Check sheet for the modelled part. Datum: model origin and axes. Units: mm. A direction names the side the tool comes from. Coordinates: 2 decimals unless noted, no trailing zeros. Write each loop counter-clockwise with the first axis right and the second up, starting at its lowest first coordinate (ties: lowest second). Pieces come first, ordered by that corner, then holes. Notation, with made-up numbers: M -19.5,12 L 21.5,12 A10 ccw 21.5,25 Z; hole C 44,-13 d8. An arc over 180 degrees is marked long. Answer as CSV lines item,"result". Start each with the question number.
1) Go/stop test with flat-tipped pins: pin 1 Ø4 at (x, z) = (4, -57.5) entering from +Y; pin 2 Ø1 at (x, y) = (0, -1) entering from +Z; pin 3 Ø0.6 at (x, z) = (0, -37) entering from +Y; pin 4 Ø4 at (x, y) = (3.5, -4) entering from -Z. Record where each tip stops, or that it passes through.
2) Material ranges on L1, parallel to X at y = 0, z = 2.5 (3 decimals); L2, parallel to Z at x = -4.25, y = 1; L3, parallel to X at y = 0.5, z = -12, recorded low to high. Write a range as [from, to].
3) Access from +Z, -Z, +X, -X, +Y, -Y to the whole of each face (thin tool, end or side, straight path). Record for faces 3 (the flat face through (0, 1.568, 3)), 4 (the cylindrical face through (0.328, -1.475, -5.759)), 5 (the flat face through (0, 4.743, -1)).
4) Section check D-D (y = -2.75). Record the cut outline in (x, z), and give its area (3 significant figures).
5) Section check C-C (z = -54.5). Record the cut outline in (x, y).
6) Section check A-A (x = 0). Record the cut outline in (y, z) (3 decimals).
7) Section check B-B (y = 0). Record the cut outline in (x, z) (3 decimals).
8) Draft check along X on faces 1 (the flat face through (1.2, -1.2, -8.89)), 2 (the cylindrical face through (0, -2, 3)). Enter one of: +X half, -X half, draft (parallel to the pull), parting line (faces both ways), or undercut.
from build123d import *

# Parameters (mm, degrees)
BOSS_EXTRUDE1_DEPTH = 6.35
BOSS_EXTRUDE2_START = 2.54
BOSS_EXTRUDE2_DEPTH = 2.54
BOSS_EXTRUDE4_START = 6.35
SKETCH4_R           = 1.5113
BOSS_EXTRUDE4_DEPTH = 6.35
BOSS_EXTRUDE3_DEPTH = 63.5


with BuildPart() as part:
    # Sketch1 → Boss-Extrude1 (new body)
    with BuildSketch(Plane.XY):
        with BuildLine():
            Line((-2.069463106, 4.743200128), (2.069463106, 4.743200128))
            ThreePointArc((2.069463106, 4.743200128), (0, -5.175), (-2.069463106, 4.743200128))
        make_face()
        with BuildLine():
            Line((-1.24126885, 1.568200128), (1.24126885, 1.568200128))
            ThreePointArc((1.24126885, 1.568200128), (0, -2), (-1.24126885, 1.568200128))
        make_face(mode=Mode.SUBTRACT)
    extrude(amount=BOSS_EXTRUDE1_DEPTH)

    # Sketch3 → Boss-Extrude2 (add)
    with BuildSketch(Plane(origin=(0, 0, 0), x_dir=(-1, 0, 0), z_dir=(0, 0, -1)).offset(BOSS_EXTRUDE2_START)):
        with BuildLine():
            Line((-2.069463106, 4.743200128), (2.069463106, 4.743200128))
            ThreePointArc((2.069463106, 4.743200128), (0, -5.175), (-2.069463106, 4.743200128))
        make_face()
    extrude(amount=-BOSS_EXTRUDE2_DEPTH)

    # Sketch4 → Boss-Extrude4 (add)
    with BuildSketch(Plane(origin=(0, 0, -2.54), x_dir=(-1, 0, 0), z_dir=(0, 0, -1)).offset(BOSS_EXTRUDE4_START)):
        with BuildLine():
            Line((2.069463106, 4.743200128), (-2.069463106, 4.743200128))
            ThreePointArc((-2.069463106, 4.743200128), (0, -5.175), (2.069463106, 4.743200128))
        make_face()
        Circle(SKETCH4_R, mode=Mode.SUBTRACT)
    extrude(amount=-BOSS_EXTRUDE4_DEPTH)

    # Sketch2 → Boss-Extrude3 (add)
    with BuildSketch(Plane(origin=(0, 0, -2.54), x_dir=(-1, 0, 0), z_dir=(0, 0, -1))):
        with BuildLine():
            Line((0.997718624, 0.892386667), (-0.997718624, 0.892386667))
            ThreePointArc((-0.997718624, 0.892386667), (0, -1.33858), (0.997718624, 0.892386667))
        make_face()
    extrude(amount=BOSS_EXTRUDE3_DEPTH)


solid = part.part
Results found:
1,pin 1,"passes through"
1,pin 2,"stops at z = 0"
1,pin 3,"stops at y = 0.89"
1,pin 4,"stops at z = -8.89"
2,L1,"x = [-5.175, -2], [2, 5.175]"
2,L2,"z = [-8.89, 6.35]"
2,L3,"x = [-1.24, 1.24]"
3,face 3,"+Z"
3,face 4,"-Z"
3,face 5,"+Z, -Z, +X, -X, +Y"
4,outline,"M -4.38,-8.89 L 4.38,-8.89 L 4.38,6.35 L -4.38,6.35 Z"
4,area,"134 mm2"
5,outline,"M -1,0.89 A1.34 ccw long 1,0.89 Z"
6,outline,"M -5.175,-8.89 L -1.511,-8.89 L -1.511,-2.54 L -1.339,-2.54 L -1.339,-66.04 L 0.892,-66.04 L 0.892,-2.54 L 1.511,-2.54 L 1.511,-8.89 L 4.743,-8.89 L 4.743,6.35 L 1.568,6.35 L 1.568,0 L -2,0 L -2,6.35 L -5.175,6.35 Z"
7,outline,"M -5.175,-8.89 L -1.511,-8.89 L -1.511,-2.54 L -1.339,-2.54 L -1.339,-66.04 L 1.339,-66.04 L 1.339,-2.54 L 1.511,-2.54 L 1.511,-8.89 L 5.175,-8.89 L 5.175,6.35 L 2,6.35 L 2,0 L -2,0 L -2,6.35 L -5.175,6.35 Z"
8,face 1,"draft"
8,face 2,"undercut"
